from build123d import *

# Parameters (mm, degrees)
SKETCH1_W           = 300
SKETCH1_H           = 88.48
SKETCH1_W_2         = 36
SKETCH1_H_2         = 36
BOSS_EXTRUDE1_DEPTH = 3


with BuildPart() as part:
    # Sketch1 → Boss-Extrude1 (new body)
    with BuildSketch(Plane.XY):
        Rectangle(SKETCH1_W, SKETCH1_H)
        with Locations((-56, 0)):
            Rectangle(SKETCH1_W_2, SKETCH1_H_2, mode=Mode.SUBTRACT)
        with Locations((-112, 0)):
            Rectangle(SKETCH1_W_2, SKETCH1_H_2, mode=Mode.SUBTRACT)
        Rectangle(SKETCH1_W_2, SKETCH1_H_2, mode=Mode.SUBTRACT)
        with Locations((56, 0)):
            Rectangle(SKETCH1_W_2, SKETCH1_H_2, mode=Mode.SUBTRACT)
        with Locations((112, 0)):
            Rectangle(SKETCH1_W_2, SKETCH1_H_2, mode=Mode.SUBTRACT)
    extrude(amount=BOSS_EXTRUDE1_DEPTH)


solid = part.part
The listing builds one solid part. Answer for the finished solid, in the listing's coordinates (mm). Give positions to 0.01 mm unless a question says otherwise; leave off trailing zeros. Write each loop counter-clockwise with the first axis right and the second up, starting at its lowest first coordinate (ties: lowest second). Pieces come first, ordered by that corner, then holes.
Item 1: Section A-A, the plane x = -1 is taken. Write down the section's boundary in (y, z).
Item 2: Find the intervals of material crossed by line 1 along X through (y, z) = (-5, 0.65); line 2 along Y through (x, z) = (-121.5, 2.7), in increasing order.
Item 3: Section C-C, the plane z = 1.8 is taken. Write down the section's boundary in (x, y).
Item 4: Section B-B, the plane y = 4.5 is taken. Write down the section's boundary in (x, z).
Completed:
1. outline: (-44.24, 0) - (-18, 0) - (-18, 3) - (-44.24, 3) - close; (18, 0) - (44.24, 0) - (44.24, 3) - (18, 3) - close
2. line 1: x = -150 to -130, -94 to -74, -38 to -18, 18 to 38, 74 to 94, 130 to 150
2. line 2: y = -44.24 to -18, 18 to 44.24
3. outline: (-150, -44.24) - (150, -44.24) - (150, 44.24) - (-150, 44.24) - close; hole (-130, -18) - (-94, -18) - (-94, 18) - (-130, 18) - close; hole (-74, -18) - (-38, -18) - (-38, 18) - (-74, 18) - close; hole (-18, -18) - (18, -18) - (18, 18) - (-18, 18) - close; hole (38, -18) - (74, -18) - (74, 18) - (38, 18) - close; hole (94, -18) - (130, -18) - (130, 18) - (94, 18) - close
4. outline: (-150, 0) - (-130, 0) - (-130, 3) - (-150, 3) - close; (-94, 0) - (-74, 0) - (-74, 3) - (-94, 3) - close; (-38, 0) - (-18, 0) - (-18, 3) - (-38, 3) - close; (18, 0) - (38, 0) - (38, 3) - (18, 3) - close; (74, 0) - (94, 0) - (94, 3) - (74, 3) - close; (130, 0) - (150, 0) - (150, 3) - (130, 3) - close
